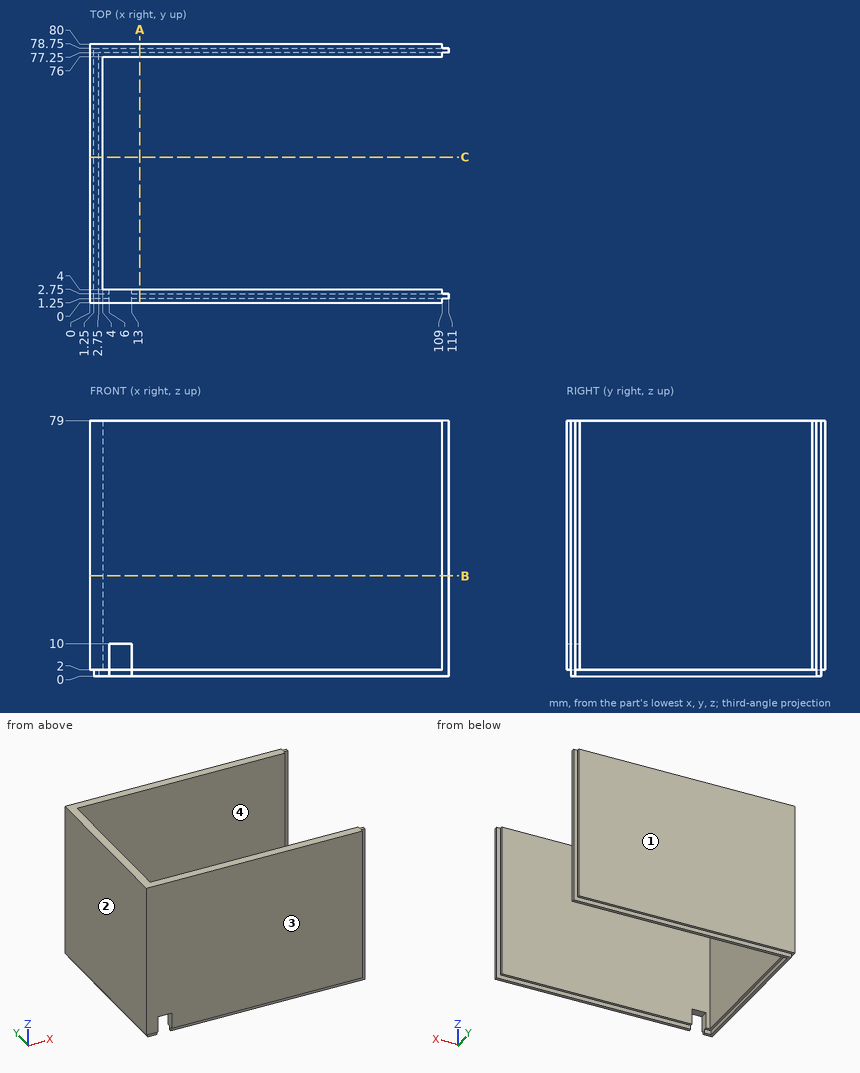
The figure shows three views and two pictorial views of one solid part (mm, origin at its lowest corner). Answer the questions. Give positions to 0.01 mm unless a question says otherwise; leave off trailing zeros. Order: outer loops, then holes, each group sorted by start corner. A loop starts at its lowest first (then second) coordinate and runs counter-clockwise, first axis right, second up. Notation, with made-up numbers: M -28.5,18.25 L -3.5,18.25 A7 cw -3.5,22.25 Z; hole C 2.25,83.5 d9. An arc over 180 degrees is marked long. Return JSON: item names as keys, results as strings.
Q1. Find section A-A, the plane x = 15.5. Write down the section's boundary in (y, z), and give its area (3 significant figures).
Answer below:
{"outline": "M 0,2 L 1.25,2 L 1.25,0 L 2.75,0 L 2.75,2 L 4,2 L 4,79 L 0,79 Z; M 76,2 L 77.25,2 L 77.25,0 L 78.75,0 L 78.75,2 L 80,2 L 80,79 L 76,79 Z", "area": "622 mm^2"}
Q2. Find section B-B, the plane z = 31. Write down the section's boundary in (x, y).
Answer below:
{"outline": "M 0,0 L 109,0 L 109,1.25 L 111,1.25 L 111,2.75 L 109,2.75 L 109,4 L 4,4 L 4,76 L 109,76 L 109,77.25 L 111,77.25 L 111,78.75 L 109,78.75 L 109,80 L 0,80 Z"}
Q3. The mould has two halves that part along Y. Classify the marked faces 1, 2, 3 and 4: pulls with the +Y half, pulls with the -Y half, needs draft (parallel to the pull), parting line crosses it, or undercut.
Answer below:
{"face 1": "pulls with the +Y half", "face 2": "needs draft", "face 3": "pulls with the -Y half", "face 4": "undercut"}
Q4. Find the intervals of material crossed by line 1 along Y through (x, z) = (80, 65.5); line 2 along X through (y, z) = (54.5, 43); line 3 along Y through (x, z) = (10, 4.5), in increasing order. Write a range as [from, to].
Answer below:
{"line 1": "y = [0, 4], [76, 80]", "line 2": "x = [0, 4]", "line 3": "y = [76, 80]"}
Q5. Find section C-C, the plane y = 45. Write down the section's boundary in (x, z).
Answer below:
{"outline": "M 0,2 L 1.25,2 L 1.25,0 L 2.75,0 L 2.75,2 L 4,2 L 4,79 L 0,79 Z"}
Q6. Each of these flat-tipped pins is pushed along its axis until it touches: pin 1 (1.6 mm diameter, centred on x = 4.5, z = 1, fed in from -Y); pin 2 (3 mm diameter, centred on x = 9, y = 2, fed in from -Z); pin 3 (12 mm diameter, centred on y = 63, z = 29.5, fed in from +X). Where does it stop, or does it pass through?
Answer below:
{"pin 1": "stops at y = 1.25", "pin 2": "stops at z = 10", "pin 3": "stops at x = 4"}
